from build123d import *

# Parameters (mm, degrees)
SKETCH_1_R          = 3
SKETCH_1_R_2        = 1.55
EXTRUDE_1_DEPTH     = 2
EXTRUDE_1_2_DEPTH   = 2
SKETCH_1_R_3        = 5.5
SKETCH_1_R_4        = 1.5
EXTRUDE_1_3_DEPTH   = 2
EXTRUDE_2_DEPTH     = 2
SKETCH_3_R          = 3
CUT_EXTRUDE_1_DEPTH = 1
FILLET_2_R          = 2
CHAMFER_1_SIZE      = 0.25
CHAMFER_1_SIZE2     = 0.144337567


with BuildPart() as part:
    # Sketch 1 → Extrude 1 (new body)
    with BuildSketch(Plane.XY):
        with Locations((5.814342437, 15.974774553)):
            Circle(SKETCH_1_R)
        with Locations((5.814342437, 15.974774553)):
            Circle(SKETCH_1_R_2, mode=Mode.SUBTRACT)
    extrude(amount=EXTRUDE_1_DEPTH)



with BuildPart() as body_2:
    # Sketch 1 → Extrude 1 2 (new body)
    with BuildSketch(Plane.XY):
        with Locations(Location((5.814342437, -15.974774553, 0), (0, 0, 180))):
            Circle(SKETCH_1_R)
        with Locations(Location((5.814342437, -15.974774553, 0), (0, 0, 180))):
            Circle(SKETCH_1_R_2, mode=Mode.SUBTRACT)
    extrude(amount=EXTRUDE_1_2_DEPTH)


with BuildPart() as body_3:
    # Sketch 1 → Extrude 1 3 (new body)
    with BuildSketch(Plane.XY):
        with BuildLine():
            ThreePointArc((3.714381625, -6.515625), (7.5, 0), (3.714381625, 6.515625))
            ThreePointArc((3.714381625, 6.515625), (0, 12), (-3.714381625, 6.515625))
            ThreePointArc((-3.714381625, 6.515625), (-7.5, 0), (-3.714381625, -6.515625))
            ThreePointArc((-3.714381625, -6.515625), (0, -12), (3.714381625, -6.515625))
        make_face()
        Circle(SKETCH_1_R_3, mode=Mode.SUBTRACT)
        with Locations((0, -8)):
            Circle(SKETCH_1_R_4, mode=Mode.SUBTRACT)
        with Locations(Location((0, 8, 0), (0, 0, 180))):
            Circle(SKETCH_1_R_4, mode=Mode.SUBTRACT)
    extrude(amount=EXTRUDE_1_3_DEPTH)


with BuildPart() as part_1:
    add(part.part)

    add(body_2.part)  # Extrude 2 merges body 2

    add(body_3.part)  # Extrude 2 merges body 3
    # Sketch 2 → Extrude 2 (add, through all)
    with BuildSketch(Plane.XY.offset(2)):
        with BuildLine():
            Line((4.046944512, 13.550665526), (2.356530565, 11.23214537))
            ThreePointArc((2.356530565, 11.23214537), (3.112774512, 10.512097697), (3.65688802, 9.620854717))
            Line((3.65688802, 9.620854717), (6.113074488, 12.98968508))
            ThreePointArc((6.113074488, 12.98968508), (5.028263798, 13.079592284), (4.046944512, 13.550665526))
        make_face()
        with BuildLine():
            ThreePointArc((0.424742649, 11.977385282), (1.439692955, 11.731927678), (2.356530565, 11.23214537))
            Line((2.356530565, 11.23214537), (4.046944512, 13.550665526))
            ThreePointArc((4.046944512, 13.550665526), (3.2983125, 14.340885525), (2.880929118, 15.346215646))
            Line((2.880929118, 15.346215646), (0.424742649, 11.977385282))
        make_face()
        with BuildLine():
            ThreePointArc((3.65688802, -9.620854717), (2.356530565, -11.23214537), (0.424742649, -11.977385282))
            Line((0.424742649, -11.977385282), (2.880929118, -15.346215646))
            ThreePointArc((2.880929118, -15.346215646), (4.046944512, -13.550665526), (6.113074488, -12.98968508))
            Line((6.113074488, -12.98968508), (3.65688802, -9.620854717))
        make_face()
    extrude(amount=-EXTRUDE_2_DEPTH)

    # Sketch 3 → Cut-Extrude 1 (cut)
    with BuildSketch(Plane.XY.offset(2)):
        with Locations((0, 8)):
            Circle(SKETCH_3_R)
        with Locations((0, -8)):
            Circle(SKETCH_3_R)
    extrude(amount=-CUT_EXTRUDE_1_DEPTH, mode=Mode.SUBTRACT)

    # Fillet 2
    fillet_2_edges = [part_1.edges().sort_by_distance(p)[0] for p in [
        (2.880929118, 15.346215646, 1),
        (6.113074488, 12.98968508, 1),
        (3.65688802, 9.620854717, 1),
        (0.424742649, 11.977385282, 1),
        (2.880929118, -15.346215646, 1),
        (0.424742649, -11.977385282, 1),
        (3.65688802, -9.620854717, 1),
        (6.113074488, -12.98968508, 1),
        (-1.36421552, 5.328125, 1.5),
        (1.36421552, 5.328125, 1.5),
        (3.714381625, 6.515625, 1),
        (1.36421552, -5.328125, 1.5),
        (3.714381625, -6.515625, 1),
        (-1.36421552, -5.328125, 1.5),
        (-3.714381625, -6.515625, 1),
        (-3.714381625, 6.515625, 1),
    ]]
    fillet(fillet_2_edges, radius=FILLET_2_R)

    # Chamfer 1
    chamfer_1_edges = [part_1.edges().sort_by_distance(p)[0] for p in [
        (-2.622819565, 5.462987902, 2),
        (-2.622819565, -5.462987902, 2),
        (2.622819565, 5.462987902, 2),
        (2.622819565, -5.462987902, 2),
        (0, -11, 2),
        (4.932006961, 2.434195419, 2),
        (-5.5, 0, 2),
        (0, 11, 2),
    ]]
    chamfer_1_side = [part_1.faces().sort_by_distance(p)[0] for p in [
        (7.086923001, 0, 2),
    ]]
    chamfer(chamfer_1_edges, length=CHAMFER_1_SIZE, length2=CHAMFER_1_SIZE2, reference=chamfer_1_side[0])


solid = part_1.part
The listing builds one solid part. Answer for the finished solid, in the listing's coordinates (mm). A direction names the side the tool comes from. Coordinates: 2 decimals unless noted, no trailing zeros. Loops run counter-clockwise (first coordinate to the right, second up) from the corner with the lowest first, then second, coordinate; pieces in that order, holes last.
1) Find section C-C on z = 1.35. Give the number of separate pieces and of enclosed holes in the cut face, then the cut area to 3 significant figures.
2) Determine the mould class of faces 1 (the face through (-3.071, 10.564, 0.986)), 2 (the face through (4.266, 16.043, 0.986)), 3 (the face through (0.325, 9.464, 0.493)), 4 (the face through (7.51, -18.45, 0.99)) for opening direction X: pulls with the +X half, pulls with the -X half, needs draft (parallel to the pull), parting line crosses it, or undercut.
3) Find section A-A on y = -8. Write down the section's boundary in (x, z).
4) Find the intervals of material crossed by L1, parallel to X at y = -8, z = 0.2; L2, parallel to X at y = -8, z = 1.6; L3, parallel to Y at x = 0, z = 0.35, in increasing order.
5) A flat-ended cylindrical pin translates along its axis: pin 1 Ø5.5 at (x, y) = (0, -7.5) entering from +Z. Find the tip coordinate at first contact, or state that the pin passes through.
6) A tool of negligible diameter and unlimited length cuts with its end or side. For faces 5 (the face through (4.947, 11.39, 1.014)), 6 (the face through (-7.5, 0.1, 1)), 7 (the face through (0.1, 11, 1.4)), from which of +Z, -Z, +X, -X, +Y, -Y can it reach the whole face along a straight path? Write none if from no direction.
7) Find section B-B on x = 0. Write down the section's boundary in (y, z).
Values:
1. separate pieces: 1
1. enclosed holes: 3
1. area: 156 mm2
2. face 1: pulls with the -X half
2. face 2: undercut
2. face 3: undercut
2. face 4: parting line crosses it
3. outline: (-4, 0) - (-1.5, 0) - (-1.5, 1) - (-3, 1) - (-3, 1.86) - (-3.25, 2) - (-4, 2) - close; (1.5, 0) - (4, 0) - (4, 2) - (3.25, 2) - (3, 1.86) - (3, 1) - (1.5, 1) - close
4. L1: x = -4 to -1.5, 1.5 to 4
4. L2: x = -4 to -3, 3 to 4
4. L3: y = -12.06 to -9.5, -6.5 to -5.5, 5.5 to 6.5, 9.5 to 12.06
5. pin 1: stops at z = 1
6. face 5: +Z, -Z, +X
6. face 6: +Z, -Z, -X
6. face 7: +Z
7. outline: (-12.06, 0) - (-9.5, 0) - (-9.5, 1) - (-11, 1) - (-11, 1.86) - (-11.25, 2) - (-12.06, 2) - close; (-6.5, 0) - (-5.5, 0) - (-5.5, 1) - (-6.5, 1) - close; (5.5, 0) - (6.5, 0) - (6.5, 1) - (5.5, 1) - close; (9.5, 0) - (12.06, 0) - (12.06, 2) - (11.25, 2) - (11, 1.86) - (11, 1) - (9.5, 1) - close
